```python
from build123d import *

# Parameters (mm, degrees)
SKETCH1_R           = 3.225
BOSS_EXTRUDE1_DEPTH = 50.8
SKETCH2_W           = 254
SKETCH2_H           = 19.05
CUT_EXTRUDE1_DEPTH  = 66.440170121
CUT_EXTRUDE4_DEPTH  = 10
SKETCH3_R           = 7.75
CUT_EXTRUDE2_DEPTH  = 58.086264546
SKETCH4_R           = 7.75
CUT_EXTRUDE3_DEPTH  = 58.086264546


with BuildPart() as part:
    # Sketch1 → Boss-Extrude1 (new body)
    with BuildSketch(Plane(origin=(0, 0, 0), x_dir=(1, 0, 0), z_dir=(0, 1, 0))):
        with BuildLine():
            Line((7.577091102, 7.577091102), (0, 15.154182204))
            Line((0, 15.154182204), (0, 18.154182204))
            ThreePointArc((0, 18.154182204), (0.75, 19.45322031), (2.25, 19.45322031))
            Line((2.25, 19.45322031), (8.985991487, 15.564193812))
            ThreePointArc((8.985991487, 15.564193812), (13.767337689, 11.552167977), (16.888139781, 6.146780193))
            Line((16.888139781, 6.146780193), (30.200329071, -30.428159285))
            ThreePointArc((30.200329071, -30.428159285), (27.555628359, -36.099738267), (21.884049378, -33.455037554))
            Line((21.884049378, -33.455037554), (14.874746988, -14.197137512))
            ThreePointArc((14.874746988, -14.197137512), (13.978238272, -13.300628796), (12.715208057, -13.411129621))
            Line((12.715208057, -13.411129621), (2.25, -19.45322031))
            ThreePointArc((2.25, -19.45322031), (0.75, -19.45322031), (0, -18.154182204))
            Line((0, -18.154182204), (0, -15.154182204))
            Line((0, -15.154182204), (7.577091102, -7.577091102))
            ThreePointArc((7.577091102, -7.577091102), (10.715625, 0), (7.577091102, 7.577091102))
        make_face()
        with Locations(Location((26.042189225, -31.94159842, 0), (0, 0, 270))):
            Circle(SKETCH1_R, mode=Mode.SUBTRACT)
        with Locations(Location((19.543806501, -14.087438625, 0), (0, 0, 270))):
            Circle(SKETCH1_R, mode=Mode.SUBTRACT)
    extrude(amount=BOSS_EXTRUDE1_DEPTH)

    # Sketch2 → Cut-Extrude1 (cut, through all)
    with BuildSketch(Plane(origin=(8.985991487, 0, 15.564193812), x_dir=(0.8660254037844355, 0, -0.5000000000000056), z_dir=(0.5000000000000056, 0, 0.8660254037844356))):
        with Locations((-1.735962308, 41.275)):
            Rectangle(SKETCH2_W, SKETCH2_H)
        with Locations((-1.735962308, 9.525)):
            Rectangle(SKETCH2_W, SKETCH2_H)
    extrude(amount=CUT_EXTRUDE1_DEPTH, mode=Mode.SUBTRACT)

    # Sketch5 → Cut-Extrude4 (cut)
    with BuildSketch(Plane(origin=(8.985991487, 0, 15.564193812), x_dir=(0.8660254037844355, 0, -0.5000000000000057), z_dir=(0.5000000000000056, 0, 0.8660254037844354))):
        Polygon((4.306128381, 7), (-7.778052996, 7), (-10.778052996, 7), (-10.778052996, 43.8), (-7.778052996, 43.8), (4.306128381, 43.8), align=None)
    extrude(amount=-CUT_EXTRUDE4_DEPTH, mode=Mode.SUBTRACT)

    # Sketch3 → Cut-Extrude2 (cut, through all)
    with BuildSketch(Plane(origin=(0, 31.75, 0), x_dir=(1, 0, 0), z_dir=(0, 1, 0))):
        with Locations((19.543806501, -14.087438625)):
            Circle(SKETCH3_R)
    extrude(amount=CUT_EXTRUDE2_DEPTH, mode=Mode.SUBTRACT)

    # Sketch4 → Cut-Extrude3 (cut, through all)
    with BuildSketch(Plane.XZ.offset(-19.05)):
        with Locations((19.543806501, 14.087438625)):
            Circle(SKETCH4_R)
    extrude(amount=CUT_EXTRUDE3_DEPTH, mode=Mode.SUBTRACT)


solid = part.part
```
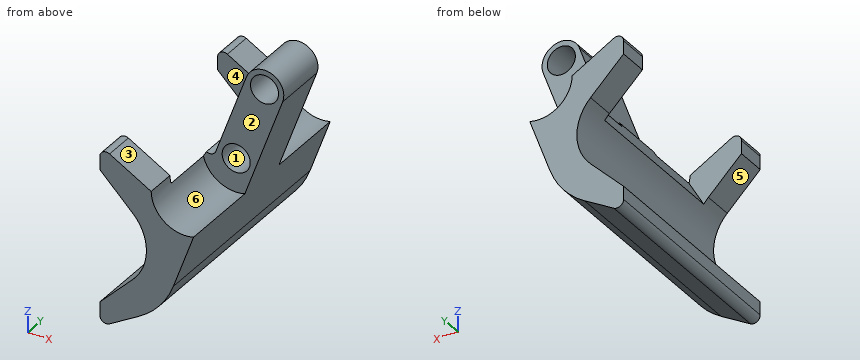
Check sheet for the modelled part. Datum: model origin and axes. Units: mm. Face numbers are marked on the shaded views. A direction names the side the tool comes from. Coordinates: 2 decimals unless noted, no trailing zeros. Write each loop counter-clockwise with the first axis right and the second up, starting at its lowest first coordinate (ties: lowest second). Pieces come first, ordered by that corner, then holes. Notation, with made-up numbers: (19.25, 24.5) -> (61.25, 24.5) arc R8 cw to (61.25, 34.5) -> close; hole circle Ø11 at (83.25, 3). An arc over 180 degrees is marked (long way). Use a Markdown table: item, result.
1. Sectioned sample at C-C (y = 4.5). Enter the section's corners in (x, z), plus the area to 3 significant figures.
Reported:
| item | result |
|---|---|
| outline | (0, -18.15) arc R1.5 ccw to (2.25, -19.45) -> (8.99, -15.56) arc R17.97 ccw to (16.89, -6.15) -> (21.53, 6.6) arc R7.75 cw to (11.8, 13.94) -> (2.25, 19.45) arc R1.5 ccw to (0, 18.15) -> (0, 15.15) -> (7.58, 7.58) arc R10.72 cw to (7.58, -7.58) -> (0, -15.15) -> close |
| area | 328 mm2 |
2. Sectioned sample at A-A (x = 6). Enter the section's corners in (y, z).
Reported:
| item | result |
|---|---|
| outline | (0, -17.29) -> (50.8, -17.29) -> (50.8, -9.15) -> (0, -9.15) -> close; (0, 9.15) -> (7, 9.15) -> (7, 17.29) -> (0, 17.29) -> close; (43.8, 9.15) -> (50.8, 9.15) -> (50.8, 17.29) -> (43.8, 17.29) -> close |
3. Release check for a two-part mould opening along Z. For the marked faces 1, 2 and 3 record: pulls with the +Z half, pulls with the -Z half, needs draft (parallel to the pull), parting line crosses it, or undercut.
Reported:
| item | result |
|---|---|
| face 1 | undercut |
| face 2 | needs draft |
| face 3 | pulls with the +Z half |
4. Sectioned sample at B-B (x = 27). Enter the section's corners in (y, z).
Reported:
| item | result |
|---|---|
| outline | (19.05, 21.64) -> (31.75, 21.64) -> (31.75, 28.86) -> (19.05, 28.86) -> close; (19.05, 35.02) -> (31.75, 35.02) -> (31.75, 36.26) -> (19.05, 36.26) -> close |
5. Go/stop test with flat-tipped pins: pin 1 Ø10.5 at (x, z) = (26.04, 31.94) entering from +Y; pin 2 Ø5 at (x, y) = (5, 30.5) entering from +Z; pin 3 Ø5 at (y, z) = (23, 27) entering from +X; pin 4 Ø8 at (x, z) = (4.5, -9.5) entering from +Y. Record where each tip stops, or that it passes through.
Reported:
| item | result |
|---|---|
| pin 1 | stops at y = 31.75 |
| pin 2 | stops at z = -7.65 |
| pin 3 | stops at x = 29.86 |
| pin 4 | stops at y = 50.8 |
6. Tool access check on the marked faces 4, 5 and 6. Record the directions out of +Z, -Z, +X, -X, +Y, -Y that give a thin tool (end or side, any length) a straight path to the whole face; none if there is none.
Reported:
| item | result |
|---|---|
| face 4 | +Z, -X |
| face 5 | -X, +Y, -Y |
| face 6 | +Z, -Y |
7. Scan lines: line 1 along Y through (x, z) = (24.5, 28.5); line 2 along X through (y, z) = (29, 30.5); line 3 along X through (y, z) = (22, -6). Record each from-to range of solid material in increasing order.
Reported:
| item | result |
|---|---|
| line 1 | y = 19.05 to 31.75 |
| line 2 | x = 20.81 to 23.16, 28.93 to 30.23 |
| line 3 | x = 8.88 to 16.94 |
8. Sectioned sample at D-D (z = 16.5). Enter the section's corners in (x, y), plus the area to 3 significant figures.
Reported:
| item | result |
|---|---|
| outline | (0, 0) -> (7.37, 0) -> (7.37, 7) -> (0, 7) -> close; (0, 43.8) -> (7.37, 43.8) -> (7.37, 50.8) -> (0, 50.8) -> close; (15.71, 19.05) -> (17.4, 19.05) -> (17.4, 31.75) -> (15.71, 31.75) -> close; (21.68, 19.05) -> (25.13, 19.05) -> (25.13, 31.75) -> (21.68, 31.75) -> close |
| area | 168 mm2 |
